from build123d import *

# Parameters (mm, degrees)
F1_DEPTH = 50.8
F2_T     = -4.7625
F3_DEPTH = 4.7625
F4_W     = 68.2625
F4_H     = 68.2625
F4_R     = 2.15265
F4_W_2   = 50.8
F4_H_2   = 50.8
F4_W_3   = 41.4684797912
F4_H_3   = 41.275
F5_DEPTH = 4.7625
F6_W     = 68.2625
F6_H     = 68.2625
F6_R     = 2.15265
F6_W_2   = 41.275
F6_H_2   = 41.275
F7_DEPTH = 4.7625
F8_R     = 2.15265
F9_DEPTH = 74.6135


# Not quite as in the source:
# - a feature names something its author has since deleted; it is built from what else it names


with BuildPart() as f1:
    # F0 (on Top) → F1 (new body)
    with BuildSketch(Plane.XY):
        with BuildLine():
            ThreePointArc((13.49375, -13.49375), (3.9522278714, -9.5415221286), (0, 0))
            Line((0, 0), (0, 1.5875))
            Line((0, 1.5875), (-50.8, 1.5875))
            Line((-50.8, 1.5875), (-50.8, 0))
            ThreePointArc((-50.8, 0), (-31.9687966129, -45.4625466129), (13.49375, -64.29375))
            Line((13.49375, -64.29375), (15.08125, -64.29375))
            Line((15.08125, -64.29375), (15.08125, -13.49375))
            Line((15.08125, -13.49375), (13.49375, -13.49375))
        make_face()
    extrude(amount=F1_DEPTH)

    # F2
    f2_openings = [f1.faces().sort_by_distance(p)[0] for p in [
        (-25.4, 1.5875, 25.4),
    ]]
    offset(amount=F2_T, openings=f2_openings)

    # F3 (cut, through all): a face of the model
    f3_faces = [f1.faces().sort_by_distance(p)[0] for p in [
        (10.31875, -38.7122831446, 25.4),
    ]]
    extrude(f3_faces, amount=-F3_DEPTH, mode=Mode.SUBTRACT)

    # F4 (on face) → F5 (join)
    with BuildSketch(Plane.YZ.offset(15.08125)):
        with Locations((-38.7122831446, 25.4)):
            Rectangle(F4_W, F4_H)
        with Locations((-68.0810331446, -3.96875)):
            Circle(F4_R, mode=Mode.SUBTRACT)
        with Locations((-38.89375, 25.4)):
            Rectangle(F4_W_2, F4_H_2, mode=Mode.SUBTRACT)
        with Locations((-9.3435331446, -3.96875)):
            Circle(F4_R, mode=Mode.SUBTRACT)
        with Locations((-68.0810331446, 54.76875)):
            Circle(F4_R, mode=Mode.SUBTRACT)
        with Locations((-9.3435331446, 54.76875)):
            Circle(F4_R, mode=Mode.SUBTRACT)
        with Locations((-38.89375, 25.4)):
            Rectangle(F4_W_2, F4_H_2)
        with Locations((-38.7122831446, 25.4)):
            Rectangle(F4_W_3, F4_H_3, mode=Mode.SUBTRACT)
    extrude(amount=F5_DEPTH)

    # F6 (on face) → F7 (join)
    with BuildSketch(Plane(origin=(0, 1.5875, 0), x_dir=(-1, 0, 0), z_dir=(0, 1, 0))):
        with Locations((25.4, 25.4)):
            Rectangle(F6_W, F6_H)
        with Locations((-3.96875, -3.96875)):
            Circle(F6_R, mode=Mode.SUBTRACT)
        with Locations((54.76875, -3.96875)):
            Circle(F6_R, mode=Mode.SUBTRACT)
        with Locations((25.4, 25.4)):
            Rectangle(F6_W_2, F6_H_2, mode=Mode.SUBTRACT)
        with Locations((-3.96875, 54.76875)):
            Circle(F6_R, mode=Mode.SUBTRACT)
        with Locations((54.76875, 54.76875)):
            Circle(F6_R, mode=Mode.SUBTRACT)
    extrude(amount=F7_DEPTH)

    # F8 (on face) → F9 (cut, through all)
    with BuildSketch(Plane(origin=(15.08125, 0, 0), x_dir=(0, -1, 0), z_dir=(-1, 0, 0))):
        with BuildLine():
            ThreePointArc((68.0810331446, 59.53125), (64.7134370992, 51.4011539546), (72.8435331446, 54.76875))
            ThreePointArc((72.8435331446, 54.76875), (71.44862919, 58.1363460454), (68.0810331446, 59.53125))
        make_face()
        with Locations((68.0810331446, 54.76875)):
            Circle(F8_R, mode=Mode.SUBTRACT)
        with Locations((68.0810331446, 54.76875)):
            Circle(F8_R)
    extrude(amount=F9_DEPTH, mode=Mode.SUBTRACT)


solid = f1.part
Geometry: final body of the model. Coordinates: model frame, mm. A direction names the side the tool comes from. Give positions to 0.01 mm unless a question says otherwise; leave off trailing zeros. Write each loop counter-clockwise with the first axis right and the second up, starting at its lowest first coordinate (ties: lowest second). Pieces come first, ordered by that corner, then holes. Notation, with made-up numbers: (28, 6.5) -> (38, 6.5) arc R18 cw to (38, 33.5) -> close; hole circle Ø8 at (24.25, -5). An arc over 180 degrees is marked (long way). Answer in a Markdown table with one row per item.
(1) Ray query, line 1 along Z through (x, y) = (-25.5, -26); line 2 along X through (y, z) = (-7, 21); line 3 along X through (y, z) = (-13, -2.5). Return the intervals inside material, ascending. Write a range as [from, to].
Answers below:
| item | result |
|---|---|
| line 1 | [0, 4.76], [46.04, 50.8] |
| line 2 | [-50.42, -45.62], [-3.37, 1.96], [15.08, 19.84] |
| line 3 | [15.08, 19.84] |
(2) Section query A-A on z = 15. Return loops of the section in (x, y), then the cut area to 3 significant figures.
Answers below:
| item | result |
|---|---|
| outline | (-59.53, 1.59) -> (-50.8, 1.59) -> (-50.8, 0) arc R64.29 ccw to (13.49, -64.29) -> (15.08, -64.29) -> (15.08, -72.84) -> (19.84, -72.84) -> (19.84, -59.45) -> (10.32, -59.45) arc R59.53 cw to (-46.04, 0) -> (-46.04, 6.35) -> (-59.53, 6.35) -> close; (-4.76, 0) arc R18.26 ccw to (10.32, -17.98) -> (19.84, -17.98) -> (19.84, -4.58) -> (15.08, -4.58) -> (15.08, -13.49) -> (13.49, -13.49) arc R13.49 cw to (0, 0) -> (0, 1.59) -> (8.73, 1.59) -> (8.73, 6.35) -> (-4.76, 6.35) -> close |
| area | 868 mm^2 |
(3) Section query B-B on x = -9. Return loops of the section in (y, z).
Answers below:
| item | result |
|---|---|
| outline | (-60.23, 0) -> (1.59, 0) -> (1.59, -8.73) -> (6.35, -8.73) -> (6.35, 4.76) -> (-55.12, 4.76) -> (-55.12, 46.04) -> (6.35, 46.04) -> (6.35, 59.53) -> (1.59, 59.53) -> (1.59, 50.8) -> (-60.23, 50.8) -> close |
(4) Draft query along X for faces 1 (the flat face through (-59.531, 4, 25)), 2 (the flat face through (-4.762, 3, 25)), 3 (the flat face through (19.844, -39, 49)), 4 (the flat face through (17, -4.581, 25)). Return one class per face: +X half, -X half, draft (parallel to the pull), parting line (faces both ways), or undercut.
Answers below:
| item | result |
|---|---|
| face 1 | -X half |
| face 2 | undercut |
| face 3 | +X half |
| face 4 | draft |
(5) Section query D-D on y = -49. Return loops of the section in (x, z).
Answers below:
| item | result |
|---|---|
| outline | (-28.13, 0) -> (15.08, 0) -> (15.08, -8.73) -> (19.84, -8.73) -> (19.84, 4.76) -> (-20.31, 4.76) -> (-20.31, 46.04) -> (19.84, 46.04) -> (19.84, 59.53) -> (15.08, 59.53) -> (15.08, 50.8) -> (-28.13, 50.8) -> close |
(6) Section query C-C on z = 1.5. Return loops of the section in (x, y), then the cut area to 3 significant figures.
Answers below:
| item | result |
|---|---|
| outline | (-59.53, 1.59) -> (-50.8, 1.59) -> (-50.8, 0) arc R64.29 ccw to (13.49, -64.29) -> (15.08, -64.29) -> (15.08, -72.84) -> (19.84, -72.84) -> (19.84, -4.58) -> (15.08, -4.58) -> (15.08, -13.49) -> (13.49, -13.49) arc R13.49 cw to (0, 0) -> (0, 1.59) -> (8.73, 1.59) -> (8.73, 6.35) -> (-59.53, 6.35) -> close |
| area | 3,920 mm^2 |
(7) Set-up query: faces 5 (the flat face through (8.731, 4, 25)), 6 (the flat face through (-18, -31, 0)), 7 (the flat face through (-18, -31, 50.8)). Return all of +Z, -Z, +X, -X, +Y, -Y with unobstructed straight access to the full face (end or side cutting, diameter ignored); none if empty.
Answers below:
| item | result |
|---|---|
| face 5 | +Z, -Z, +X, +Y |
| face 6 | -Z, -X, -Y |
| face 7 | +Z, -X, -Y |
(8) Pin query (flat end, axial travel): pin 1 (8 mm diameter, centred on x = 6.5, z = 37.5, fed in from -Y); pin 2 (7 mm diameter, centred on y = -9.34, z = 54.77, fed in from -X); pin 3 (0.8 mm diameter, centred on y = 0.5, z = 23.5, fed in from +X). Return the tip coordinate at first contact, or that it passes through.
Answers below:
| item | result |
|---|---|
| pin 1 | y = -64.22 |
| pin 2 | x = 15.08 |
| pin 3 | x = 0 |
